```python
from build123d import *

# Parameters (mm, degrees)
F1_DEPTH = 12.7
F2_W     = 12.7
F2_H     = 12.7
F3_DEPTH = 12.7


with BuildPart() as f1:
    # F0 (on Front) → F1 (new body)
    with BuildSketch(Plane.XZ):
        Polygon((0, 38.1), (0, 0), (25.4, 0), (25.4, 25.4), (12.7, 25.4), (12.7, 38.1), align=None)
    extrude(amount=F1_DEPTH)

    # F2 (on face) → F3 (join)
    with BuildSketch(Plane(origin=(0, 0, 0), x_dir=(-1, 0, 0), z_dir=(0, 1, 0))):
        with Locations((-19.05, 6.35)):
            Rectangle(F2_W, F2_H)
    extrude(amount=F3_DEPTH)


solid = f1.part
```
Could you check a few things on this model? Use its own coordinates, in mm. A direction names the side the tool comes from. Coordinates: 2 decimals unless noted, no trailing zeros. Loops run counter-clockwise (first coordinate to the right, second up) from the corner with the lowest first, then second, coordinate; pieces in that order, holes last.
1) Imagine slicing it at A-A (z = 5.5). List the corners of the cut face in (x, y) for me.
Reported:
outline: (0, -12.7) - (25.4, -12.7) - (25.4, 12.7) - (12.7, 12.7) - (12.7, 0) - (0, 0) - close
2) Will these pins go through, and if not, where does the flat tip stop? pin 1 Ø4 at (y, z) = (-4.5, 29.5) entering from +X; pin 2 Ø2 at (x, y) = (14, 4) entering from +Z; pin 3 Ø1.5 at (x, z) = (16, 23) entering from +Y.
Reported:
pin 1: stops at x = 12.7
pin 2: stops at z = 12.7
pin 3: stops at y = 0
3) Please list where these lines run through material, in increasing order: line 1 along Y through (x, z) = (10.5, 29); line 2 along X through (y, z) = (9.75, 8); line 3 along Z through (x, y) = (14, 3.5).
Reported:
line 1: y = -12.7 to 0
line 2: x = 12.7 to 25.4
line 3: z = 0 to 12.7
4) Imagine slicing it at B-B (y = 2). List the corners of the cut face in (x, z) for me.
Reported:
outline: (12.7, 0) - (25.4, 0) - (25.4, 12.7) - (12.7, 12.7) - close
5) Imagine slicing it at C-C (x = 8). List the corners of the cut face in (y, z) for me.
Reported:
outline: (-12.7, 0) - (0, 0) - (0, 38.1) - (-12.7, 38.1) - close
6) Which directions (+Z, -Z, +X, -X, +Y, -Y) give clear straight access to the entire face, cutting with the end or side of a thin tool? Please do faces 1 (the face through (12.7, 6, 6)), 2 (the face through (19, 12.7, 6)), 3 (the face through (19, -6, 25.4)), 4 (the face through (19, 6, 12.7)).
Reported:
face 1: +Z, -Z, -X, +Y
face 2: +Z, -Z, +X, -X, +Y
face 3: +Z, +X, +Y, -Y
face 4: +Z, +X, -X, +Y
